Autodesk Inventor part; units mm, degrees
ref_plane "YZ Plane" through (0, 0, 0) normal (1, 0, 0) x (0, 1, 0)
ref_plane "XZ Plane" through (0, 0, 0) normal (0, 1, 0) x (-1, 0, 0)
ref_plane "XY Plane" through (0, 0, 0) normal (0, 0, 1) x (1, 0, 0)
sketch "Sketch1" plane through (0, 0, 0) normal (0, 1, 0) x (-1, 0, 0)
  line L0 (0, 0) -> (8, 0)
  line L1 (8, -30) -> (0, -30)
  line L2 (0, -30) -> (0, 0)
  line L3 (6.25, -3.4) -> (1.75, -3.4)
  line L4 (1.75, -3.4) -> (1.75, -6.4)
  line L5 (1.75, -6.4) -> (6.25, -6.4)
  line L6 (6.25, -6.4) -> (6.25, -3.4)
  line L7 (6.25, -23.6) -> (1.75, -23.6)
  line L8 (1.75, -23.6) -> (1.75, -26.6)
  line L9 (1.75, -26.6) -> (6.25, -26.6)
  line L10 (6.25, -26.6) -> (6.25, -23.6)
  line L11 (8, 0) -> (30, -7.5)
  line L12 (30, -7.5) -> (30, -22.5)
  line L13 (30, -22.5) -> (8, -30)
  dimension "d0" = 30
  dimension "d1" = 8
  dimension "d2" = 4.5
  dimension "d3" = 3
  dimension "d4" = 3
  dimension "d5" = 17.2
  dimension "d6" = 3.4
  dimension "d7" = 1.75
  dimension "d8" = 15
  dimension "d9" = 7.5
  dimension "d10" = 22
  dimension "d11" = 22
extrude "Extrusion1" add sketch "Sketch1" along normal blind 3
sketch "Sketch2" plane through (0, 0, 0) normal (0, -1, 0) x (1, 0, 0)
  line L0 (0, -30) -> (-8, -30)
  line L1 (0, -30) -> (-8, -30)
  line L2 (-8, -30) -> (-14.7467, -27.7)
  line L3 (-8, -30) -> (-30, -22.5)
  line L4 (-14.7467, -27.7) -> (0, -27.7)
  line L5 (0, 0) -> (0, -30)
  line L6 (0, -27.7) -> (0, -30)
  line L7 (-14.7467, -2.3) -> (-8, 0)
  line L8 (-8, 0) -> (0, 0)
  line L9 (-14.7467, -2.3) -> (0, -2.3)
  line L10 (0, 0) -> (0, -2.3)
  dimension "d14" = 2.3
  dimension "d15" = 2.3
  dimension "d26" = 14.7467
extrude "Extrusion2" add sketch "Sketch2" along normal blind 7
sketch "Sketch3" plane through (0, 0, 0) normal (0, -1, 0) x (1, 0, 0)
  line L0 (-27, -22.3) -> (-24, -22.3)
  line L1 (-24, -22.3) -> (-24, -7.7)
  line L2 (-24, -7.7) -> (-27, -7.7)
  line L3 (-27, -7.7) -> (-27, -22.3)
  line L4 (0, -2.3) -> (0, -27.7)
  circle A0 centre (-7, -15) radius 1.4
  circle A1 centre (-7, -15) radius 2
  line L5 (-8, -30) -> (0, -30)
  point P0 (0, 0)
  point P1 (-30, -7.5)
  point P2 (-30, -22.5)
  dimension "d27" = 3
  dimension "d28" = 24
  dimension "d29" = 14.6
  dimension "d30" = 0.2
  dimension "d31" = 2.8
  dimension "d32" = 4
  dimension "d33" = 7
  dimension "d34" = 15
extrude "Extrusion3" add sketch "Sketch3" along normal blind 4
fillet "Fillet1" radius 2 1 edges at (-9, 0, -15)
sketch "Sketch4" plane through (0, 3, 0) normal (0, 1, 0) x (1, 0, 0)
  circle A0 centre (-7, 15) radius 2
  circle A1 centre (-7, 15) radius 1.4
  circle A2 centre (-7, 15) radius 4
  line L0 (-1.75, 10) -> (-6.25, 10)
  line L1 (-6.25, 10) -> (-1.75, 12)
  line L2 (-1.75, 10) -> (-1.75, 12)
  line L3 (-1.75, 18) -> (-1.75, 20)
  line L4 (-1.75, 20) -> (-6.25, 20)
  line L5 (-6.25, 20) -> (-1.75, 18)
  point P0 (0, 0)
  point P1 (-6.25, 6.4)
  point P2 (-1.75, 6.4)
  point P3 (-6.25, 23.6)
  point P4 (-1.75, 23.6)
  dimension "d38" = 3
  dimension "d39" = 2
  dimension "d40" = 2
  dimension "d41" = 3
extrude "Extrusion4" cut sketch "Sketch4" against normal blind 5 contours L0 L1 L2 | L5 L4 L3
sketch "Sketch5" plane through (0, 3, 0) normal (0, 1, 0) x (1, 0, 0)
  circle A0 centre (-15.5, 17.5) radius 3
  line L0 (0, 0) -> (0, 30)
  point P0 (-30, 22.5)
  dimension "d44" = 6
  dimension "d45" = 15.5
  dimension "d46" = 5
extrude "Extrusion5" cut sketch "Sketch5" against normal blind 5
sketch "Sketch6" plane through (0, 3, 0) normal (0, 1, 0) x (1, 0, 0)
  line L0 (-6.25, 26.6) -> (-1.75, 26.6)
  line L1 (-1.75, 23.6) -> (-6.25, 23.6)
  line L2 (-6.25, 26.6) -> (-1.75, 26.6)
  line L3 (-1.75, 26.6) -> (-1.75, 23.6)
  line L4 (-1.75, 23.6) -> (-6.25, 23.6)
  line L5 (-6.25, 23.6) -> (-6.25, 26.6)
  line L6 (-6.25, 6.4) -> (-1.75, 6.4)
  line L7 (-6.25, 6.4) -> (-1.75, 6.4)
  line L8 (-1.75, 6.4) -> (-1.75, 3.4)
  line L9 (-1.75, 3.4) -> (-6.25, 3.4)
  line L10 (-6.25, 3.4) -> (-6.25, 6.4)
  line L11 (-8, 0) -> (0, 0)
  line L12 (0, 0) -> (-8, 0)
  line L13 (0, 0) -> (0, 30)
  line L14 (0, 7.5) -> (0, 0)
  line L15 (0, 30) -> (-8, 30)
  line L16 (0, 22.5) -> (0, 30)
  line L17 (-8, 30) -> (-30, 22.5)
  line L18 (-8, 30) -> (-17, 26.9318)
  line L19 (0, 22.5) -> (-17, 22.5)
  line L20 (-17, 26.9318) -> (-17, 22.5)
  line L21 (-8, 0) -> (-17, 3.0682)
  line L22 (-30, 7.5) -> (-8, 0)
  line L23 (-17, 3.0682) -> (-17, 7.5)
  line L24 (-17, 7.5) -> (0, 7.5)
  dimension "d52" = 3
  dimension "d55" = 17
  dimension "d56" = 1.1
  dimension "d57" = 17
  dimension "d58" = 1.1
extrude "Extrusion7" add sketch "Sketch6" along normal blind 13
chamfer "Chamfer1" distance 9.5 angle 45 2 edges at (-17, 16, -24.7159) (-17, 16, -5.2841)
chamfer "Chamfer2" distance 3.5 angle 45 2 edges at (-17, 6.5, -5.2841) (-17, 6.5, -24.7159)
sketch "Sketch9" plane through (0, -4, 0) normal (0, -1, 0) x (1, 0, 0)
  line L0 (-27, -22.3) -> (-24, -22.3)
  line L1 (-24, -22.3) -> (-24, -7.7)
  line L2 (-27, -22.3) -> (-24, -22.3)
  line L3 (-24, -22.3) -> (-24, -7.7)
  line L4 (-24, -7.7) -> (-27, -7.7)
  line L5 (-27, -7.7) -> (-27, -22.3)
  point P0 (0, 0)
extrude "Extrusion10" cut sketch "Sketch9" against normal blind 1
properties part number "IRMount_top"
Geometry check sheet. Reference: the model listing, model coordinates, mm. A direction names the side the tool comes from. Coordinates: 2 decimals unless noted, no trailing zeros. Order: outer loops, then holes, each group sorted by start corner. A loop starts at its lowest first (then second) coordinate and runs counter-clockwise, first axis right, second up.
Q1. Sectioned sample at D-D on x = -15.5. Record the cut outline in (y, z), and give its area (3 significant figures).
Reply:
outline: (0, -27.44) - (6.62, -27.44) - (6.62, -22.5) - (3, -22.5) - (3, -20.5) - (0, -20.5) - close; (0, -14.5) - (3, -14.5) - (3, -7.5) - (6.62, -7.5) - (6.62, -2.56) - (0, -2.56) - close
area: 92.5 mm2
Q2. Tool access check on faces 5 (the face through (-1.75, 2, -19)), 6 (the face through (-6.1, -4, -16.3)), 7 (the face through (-25, -1, -7.7)). Record the directions out of +Z, -Z, +X, -X, +Y, -Y that give a thin tool (end or side, any length) a straight path to the whole face; none if there is none.
Reply:
face 5: +Y, -Y
face 6: +X, -X, -Y
face 7: +Z, +X, -X, -Y
Q3. Draft check along X on faces 1 (the face through (-4, 16, -27)), 2 (the face through (0, 2, -15)), 3 (the face through (-8.03, -1.97, -15.95)), 4 (the face through (-27, -1, -15)). Enter one of: released by +X, released by -X, zero draft, split by the parting line, or undercut.
Reply:
face 1: zero draft
face 2: released by +X
face 3: undercut
face 4: released by -X
Q4. Thickness scan on probe 1 along Z at (x, y) = (-7, -2.3); probe 2 along Z at (x, y) = (-8, 6.75); probe 3 along X at (y, z) = (1.8, -17.5). Record the ranges inside material, lowest first.
Reply:
probe 1: z = -30 to -27.7, -17 to -16.4, -13.6 to -13, -2.3 to 0
probe 2: z = -30 to -22.5, -7.5 to 0
probe 3: x = -30 to -18.5, -12.5 to 0
Q5. Sectioned sample at A-A on y = 12.25. Record the cut outline in (x, z), and give its area (3 significant figures).
Reply:
outline: (-11.25, -28.89) - (-8, -30) - (0, -30) - (0, -22.5) - (-11.25, -22.5) - close; (-11.25, -7.5) - (0, -7.5) - (0, 0) - (-8, 0) - (-11.25, -1.11) - close; hole (-6.25, -26.6) - (-1.75, -26.6) - (-1.75, -23.6) - (-6.25, -23.6) - close; hole (-6.25, -6.4) - (-1.75, -6.4) - (-1.75, -3.4) - (-6.25, -3.4) - close
area: 138 mm2
Q6. Sectioned sample at B-B on y = 1.5. Record the cut outline in (x, z).
Reply:
outline: (-30, -22.5) - (-8, -30) - (0, -30) - (0, 0) - (-8, 0) - (-30, -7.5) - close; hole circle Ø6 at (-15.5, -17.5); hole (-6.25, -26.6) - (-1.75, -26.6) - (-1.75, -23.6) - (-6.25, -23.6) - close; hole (-6.25, -20) - (-1.75, -20) - (-1.75, -18) - close; hole (-6.25, -10) - (-1.75, -12) - (-1.75, -10) - close; hole (-6.25, -6.4) - (-1.75, -6.4) - (-1.75, -3.4) - (-6.25, -3.4) - close
Q7. Depth check by flat-ended pin: pin 1 Ø1.5 at (y, z) = (-2, -12.5) entering from +X; pin 2 Ø2 at (x, z) = (-5, -13.5) entering from -Y; pin 3 Ø8 at (x, y) = (-12.5, -0.5) entering from -Z; pin 4 Ø5 at (x, y) = (-24.5, 6) entering from -Z. Enter the tip coordinate at first touch or a pass-through.
Reply:
pin 1: stops at x = -6.03
pin 2: stops at y = -4
pin 3: stops at z = -29.83
pin 4: passes through
